For this review, use the dimensioned drawing (mm, ordinates from the lowest corner) and the shaded views. Give positions to 0.01 mm unless a question says otherwise; leave off trailing zeros. Order: outer loops, then holes, each group sorted by start corner. A loop starts at its lowest first (then second) coordinate and runs counter-clockwise, first axis right, second up. Notation, with made-up numbers: M -12,60 L 44,60 A25 cw 44,81 Z; hole C -32.5,-35.75 d3. An arc over 180 degrees is marked long. Use CSV: the item, a comma, the result in double quotes. Start each with the question number.
(1) Clearance check with flat-ended pins moving along their axes: P1, Ø2, axis at x = 45, y = 45, coming from the +Z side; P2, Ø8, axis at x = 35.5, y = 37, coming from the +Z side; P3, Ø1.5, axis at y = 53, z = 74.5, coming from the -X side. State where each tip first meets the part, or that it passes through.
(2) Consider section A-A (x = 50.8). Write out the cut boundary in (y, z).
(3) Draft analysis for pull direction Y (two halves, no side actions). For the marked faces 1, 2, 3 and 4, state which applies: pulls with the +Y half, pulls with the -Y half, needs draft (parallel to the pull), parting line crosses it, or undercut.
(4) Wall thickness on L1, parallel to Y at x = 18, z = 23.5; L2, parallel to X at y = 17.5, z = 51; L3, parallel to Z at x = 51.5, y = 53: over which ranges is each line inside the solid? List them lowest first. Write a range as from..to.
(5) Consider section C-C (y = 11). Write out the cut boundary in (x, z).
(6) Consider section D-D (y = 44.45). Write out the cut boundary in (x, z) (3 decimals).
(7) Consider section B-B (z = 50.8). Write out the cut boundary in (x, y) (3 decimals).
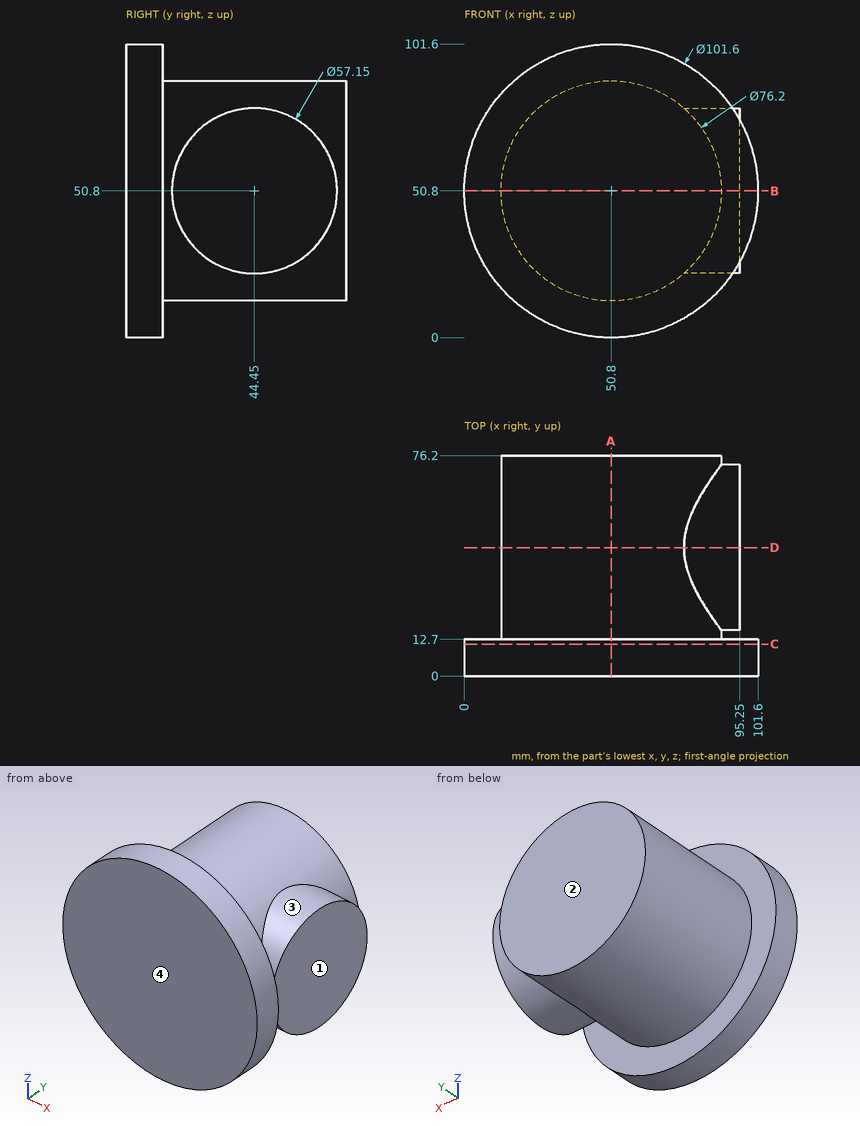
Check result:
1,P1,"stops at z = 88.6"
1,P2,"stops at z = 87.19"
1,P3,"stops at x = 20.39"
2,outline,"M 0,0 L 12.7,0 L 12.7,12.7 L 76.2,12.7 L 76.2,88.9 L 12.7,88.9 L 12.7,101.6 L 0,101.6 Z"
3,face 1,"needs draft"
3,face 2,"pulls with the +Y half"
3,face 3,"undercut"
3,face 4,"pulls with the -Y half"
4,L1,"y = 0..12.7"
4,L2,"x = 12.7..95.25"
4,L3,"z = 12.71..88.89"
5,outline,"C 50.8,50.8 d101.6"
6,outline,"M 76.001,22.225 L 95.25,22.225 L 95.25,79.375 L 76.001,79.375 A38.1 ccw long Z"
7,outline,"M 0,0 L 101.6,0 L 101.6,12.7 L 88.9,12.7 L 88.9,15.875 L 95.25,15.875 L 95.25,73.025 L 88.9,73.025 L 88.9,76.2 L 12.7,76.2 L 12.7,12.7 L 0,12.7 Z"
